For this review, take the finished solid that the model builds, in its own axes (mm). Coordinates: 2 decimals unless noted, no trailing zeros. Loops run counter-clockwise (first coordinate to the right, second up) from the corner with the lowest first, then second, coordinate; pieces in that order, holes last.
1. To check wall thickness, follow probe 1 along Z at (x, y) = (0, 1.15) (1 decimal); probe 2 along Z at (x, y) = (22, 2.95); probe 3 along Z at (x, y) = (0.5, 2.9) (3 decimals). State the ranges of each line that lie inside material, in increasing order.
2. Clearance check with flat-ended pins moving along their axes: P1, Ø1.6, axis at x = 25.5, y = 1, coming from the -Z side; P2, Ø1.6, axis at y = 1.5, z = -33.5, coming from the +X side. State where each tip first meets the part, or that it passes through.
3. Mouldability with a two-part tool opening along X and no side actions: class faces 1 (the face through (48.89, 1.61, 10.89)), 2 (the face through (32, 2, -12.7)), 3 (the face through (39.76, 1.57, -0.48)), 4 (the face through (-0.85, 1.57, -39.44)) as pulls with the +X half, pulls with the -X half, needs draft (parallel to the pull), parting line crosses it, or undercut.
4. Take a section at D-D, the plane z = 0. State the section outline as (x, y) points (1 decimal), then the cut area to 3 significant figures.
5. Take a section at A-A, the plane x = 0. State the section outline as (y, z) points (1 decimal), then the cut area to 3 significant figures.
6. Take a section at C-C, the plane z = -38.1. State the section outline as (x, y) points (1 decimal), then the cut area to 3 significant figures.
7. Take a section at B-B, the plane y = 1.85. Count the separate pieces of the cut face and the enclosed holes in it, then the cut area to 3 significant figures.
Autodesk Inventor part; units mm, degrees
ref_plane "YZ Plane" through (0, 0, 0) normal (1, 0, 0) x (0, 1, 0)
ref_plane "XZ Plane" through (0, 0, 0) normal (0, 1, 0) x (-1, 0, 0)
ref_plane "XY Plane" through (0, 0, 0) normal (0, 0, 1) x (1, 0, 0)
sketch "Sketch1" plane through (0, 0, 0) normal (0, 1, 0) x (-1, 0, 0)
  circle A0 centre (0, 0) radius 1.5875
  line L0 (0, 0) -> (0, -38.1) construction
  circle A1 centre (-22.225, 0) radius 1.5875
  circle A2 centre (-41.275, 0) radius 1.5875
  circle A3 centre (0, -19.05) radius 1.5875
  circle A4 centre (0, -38.1) radius 1.5875
  line L1 (-12.7, -12.7) -> (-50.8, -12.7)
  line L2 (-50.8, -12.7) -> (-50.8, 12.7)
  line L3 (-50.8, 12.7) -> (12.7, 12.7)
  line L4 (12.7, 12.7) -> (12.7, -47.625)
  line L5 (12.7, -47.625) -> (-12.7, -47.625)
  line L6 (-12.7, -47.625) -> (-12.7, -12.7)
  line L7 (0, -38.1) -> (0, -47.625) construction
  line L8 (-41.275, 0) -> (-50.8, 0) construction
  line L9 (-12.7, -12.7) -> (-12.7, 12.7) construction
  line L10 (0, 0) -> (-41.275, 0) construction
  dimension "d0" = 3.175
  dimension "d1" = 22.225
  dimension "d2" = 25.4
  dimension "d3" = 9.525
  dimension "d4" = 19.05
  dimension "d5" = 19.05
extrude "Extrusion1" add sketch "Sketch1" along normal blind 3.175
fillet "Fillet1" radius 6.35 6 edges at (50.8, 1.5875, 12.7) (50.8, 1.5875, -12.7) (12.7, 1.5875, -47.625) (-12.7, 1.5875, -47.625) (-12.7, 1.5875, 12.7) (12.7, 1.5875, -12.7)
properties part number "plate" material "Aluminum 6061"
Results list:
1. probe 1: z = -47.6 to -39.7, -36.5 to -20.6, -17.5 to -1.6, 1.6 to 12.7
1. probe 2: z = -12.7 to -1.57, 1.57 to 12.7
1. probe 3: z = -47.625 to -39.607, -36.593 to -20.557, -17.543 to -1.507, 1.507 to 12.7
2. P1: stops at z = -12.7
2. P2: stops at x = 12.7
3. face 1: pulls with the +X half
3. face 2: needs draft
3. face 3: undercut
3. face 4: undercut
4. outline: (-12.7, 0) - (-1.6, 0) - (-1.6, 3.2) - (-12.7, 3.2) - close; (1.6, 0) - (20.6, 0) - (20.6, 3.2) - (1.6, 3.2) - close; (23.8, 0) - (39.7, 0) - (39.7, 3.2) - (23.8, 3.2) - close; (42.9, 0) - (50.8, 0) - (50.8, 3.2) - (42.9, 3.2) - close
4. area: 171 mm2
5. outline: (0, -47.6) - (3.2, -47.6) - (3.2, -39.7) - (0, -39.7) - close; (0, -36.5) - (3.2, -36.5) - (3.2, -20.6) - (0, -20.6) - close; (0, -17.5) - (3.2, -17.5) - (3.2, -1.6) - (0, -1.6) - close; (0, 1.6) - (3.2, 1.6) - (3.2, 12.7) - (0, 12.7) - close
5. area: 161 mm2
6. outline: (-12.7, 0) - (-1.6, 0) - (-1.6, 3.2) - (-12.7, 3.2) - close; (1.6, 0) - (12.7, 0) - (12.7, 3.2) - (1.6, 3.2) - close
6. area: 70.6 mm2
7. separate pieces: 1
7. enclosed holes: 5
7. area: 2,430 mm2
